```python
from build123d import *

# Parameters (mm, degrees)
BOSS_EXTRUDE1_DEPTH = 15
CUT_EXTRUDE4_DEPTH  = 3
FILLET1_R           = 7.5


with BuildPart() as part:
    # Sketch1 → Boss-Extrude1 (new body)
    with BuildSketch(Plane(origin=(0, 0, 0), x_dir=(0, 0, -1), z_dir=(1, 0, 0))):
        with BuildLine():
            Line((105.176560834, -44.266250702), (105.176560834, -78.308566478))
            Line((105.176560834, -78.308566478), (-47.323439166, -78.308566478))
            Line((-47.323439166, -78.308566478), (-47.323439166, 41.691433522))
            Line((-47.323439166, 41.691433522), (50.746660587, 41.691433522))
            ThreePointArc((50.746660587, 41.691433522), (80.628611175, 29.313924319), (93.006120378, -0.568026269))
            Line((93.006120378, -0.568026269), (93.006120378, -20.545339005))
            ThreePointArc((93.006120378, -20.545339005), (94.435922822, -26.464268202), (98.409995921, -31.077813571))
            ThreePointArc((98.409995921, -31.077813571), (103.386206676, -36.854751618), (105.176560834, -44.266250702))
        make_face()
    extrude(amount=BOSS_EXTRUDE1_DEPTH)

    # Sketch3 → Cut-Extrude4 (cut)
    with BuildSketch(Plane(origin=(15, 0, 0), x_dir=(0, 0, -1), z_dir=(1, 0, 0))):
        Polygon((90.676560834, -71.308566478), (90.676560834, -39.308566478), (29.831261372, -39.308566478), (-10.168738628, 29.973465825), (-42.323439166, 29.973465825), (-42.323439166, -71.308566478), (-40.323439166, -71.308566478), (-40.323439166, 27.973465825), (-11.323439166, 27.973465825), (28.676560834, -41.308566478), (88.676560834, -41.308566478), (88.676560834, -71.308566478), align=None)
    extrude(amount=-CUT_EXTRUDE4_DEPTH, mode=Mode.SUBTRACT)

    # Fillet1
    fillet1_edges = [part.edges().sort_by_distance(p)[0] for p in [
        (15, 29.313924319, -80.628611175),
        (0, -10.556682637, -93.006120378),
        (0, -26.464268202, -94.435922822),
        (15, 41.691433522, -1.711610711),
        (15, -61.28740859, -105.176560834),
        (15, -36.854751618, -103.386206676),
        (15, -10.556682637, -93.006120378),
        (0, -61.28740859, -105.176560834),
        (0, 41.691433522, -1.711610711),
    ]]
    fillet(fillet1_edges, radius=FILLET1_R - 0.0001)  # a hair under: the kernel refuses the full size


solid = part.part
```
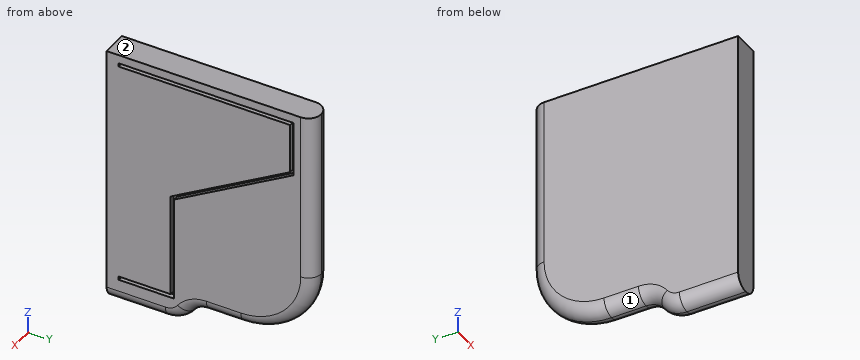
Build history of the part. All positions in model axes, mm. Face numbers are marked on the shaded views. A direction names the side the tool comes from. Give positions to 0.01 mm unless a question says otherwise; leave off trailing zeros. Loops run counter-clockwise (first coordinate to the right, second up) from the corner with the lowest first, then second, coordinate; pieces in that order, holes last.
Item 1: Which spindle directions (+Z, -Z, +X, -X, +Y, -Y) get a long thin tool onto all of the face, cutting with end or side? Do the marked faces 1 and 2. Say none if no direction does.
Answers follow:
face 1: -Z, -X, +Y
face 2: +Z, +X, -X, +Y, -Y
Item 2: Flat gauge pins, fed straight in: pin 1 (3.5 mm diameter, centred on x = 13.5, z = 28, fed in from +Y); pin 2 (2.5 mm diameter, centred on x = 14, y = -63.5, fed in from -Z); pin 3 (3.5 mm diameter, centred on x = 14, z = -63.5, fed in from +Y). Where does each tip first touch, or does it go through?
Answers follow:
pin 1: stops at y = 40.37
pin 2: stops at z = -103.03
pin 3: stops at y = 38.04
Item 3: Drill centre lines: line 1 (Z direction, x = 13.25, y = 14); line 2 (X direction, y = -34.5, z = -92); line 3 (Z direction, x = 13.25, y = 26). Where is each one in solid material? Low to high.
Answers follow:
line 1: z = -87.54 to 0.95, 3.26 to 40.32, 42.32 to 47.32
line 2: x = 0.03 to 14.97
line 3: z = -80.08 to 7.87, 10.18 to 40.32, 42.32 to 47.32
Item 4: Slice it at C-C, the plane x = 9.5. List the corners of the cut face in (y, z) (1 decimal).
Answers follow:
outline: (-78.3, -104.9) - (-44.3, -104.9) arc R16 ccw to (-31.3, -98.3) arc R13.2 cw to (-20.5, -92.7) - (-0.6, -92.7) arc R42 ccw to (41.4, -50.7) - (41.4, 47.3) - (-78.3, 47.3) - close
